For this review, take the finished solid that the model builds, in its own axes (mm). Give positions to 0.01 mm unless a question says otherwise; leave off trailing zeros. Order: outer loops, then holes, each group sorted by start corner. A loop starts at its lowest first (then second) coordinate and runs counter-clockwise, first axis right, second up. Notation, with made-up numbers: M 75.25,18 L 114.25,18 A16 cw 114.25,30 Z; hole C -31.75,11.5 d8. An arc over 180 degrees is marked long. Use CSV: the item, a comma, the result in double quotes. Start each with the question number.
(1) Wall thickness on L1, parallel to X at y = 25.5, z = 0; L2, parallel to Z at x = 0.25, y = 29.5; L3, parallel to Z at x = 0.4, y = 14: over which ranges is each line inside the solid? List them lowest first. Write a range as from..to.
(2) Consider section A-A (z = 0). Write out the cut boundary in (x, y), and give its area (3 significant figures).
(3) Draft analysis for pull direction Z (two halves, no side actions). For faces 1 (the face through (1.109, 24.653, 1.958)), 2 (the face through (-1.22, 24.65, -0.27)), 3 (the face through (-2.25, 25, 0)), state which applies: pulls with the +Z half, pulls with the -Z half, needs draft (parallel to the pull), parting line crosses it, or undercut.
(4) Consider section B-B (y = 37). Write out the cut boundary in (x, z).
(5) Clearance check with a flat-ended pin moving along its axis: P1, Ø1, axis at y = 7.5, z = 2, coming from the -X side. State where the tip first meets the part, or that it passes through.
```python
from build123d import *

# Parameters (mm, degrees)
SKETCH1_R           = 1.25
BOSS_EXTRUDE1_DEPTH = 50


with BuildPart() as part:
    # Sketch1 → Boss-Extrude1 (new body)
    with BuildSketch(Plane(origin=(0, 0, 0), x_dir=(1, 0, 0), z_dir=(0, 1, 0))):
        Polygon((0, 2.598076211), (-2.25, 1.299038106), (-2.25, -1.299038106), (0, -2.598076211), (2.25, -1.299038106), (2.25, 1.299038106), align=None)
        with Locations(Location((0, 0, 0), (0, 0, 270))):
            Circle(SKETCH1_R, mode=Mode.SUBTRACT)
    extrude(amount=BOSS_EXTRUDE1_DEPTH)

    # Sketch2 → Cut-Revolve1 (revolve, cut)
    with BuildSketch(Plane(origin=(0, 0, 0), x_dir=(0, 0, -1), z_dir=(1, 0, 0))):
        Polygon((-2.098076211, 50), (-2.598076211, 49.4), (-2.598076211, 50), align=None)
    cut_revolve1 = revolve(axis=Axis((0, 50, 0), (0, -1, 0)), mode=Mode.SUBTRACT)

    # Mirror1: Cut-Revolve1 across plane
    add(cut_revolve1.mirror(Plane.ZX.offset(25)), mode=Mode.SUBTRACT)


solid = part.part
```
Check result:
1,L1,"x = -2.25..-1.25, 1.25..2.25"
1,L2,"z = -2.45..-1.22, 1.22..2.45"
1,L3,"z = -2.37..-1.18, 1.18..2.37"
2,outline,"M -2.25,0.18 L -2.1,0 L -1.25,0 L -1.25,50 L -2.1,50 L -2.25,49.82 Z; M 1.25,0 L 2.1,0 L 2.25,0.18 L 2.25,49.82 L 2.1,50 L 1.25,50 Z"
2,area,"99.9 mm^2"
3,face 1,"pulls with the +Z half"
3,face 2,"undercut"
3,face 3,"needs draft"
4,outline,"M -2.25,-1.3 L 0,-2.6 L 2.25,-1.3 L 2.25,1.3 L 0,2.6 L -2.25,1.3 Z; hole C 0,0 d2.5"
5,P1,"stops at x = -1.9"
